from build123d import *

# Parameters (mm, degrees)
F1_DEPTH  = 101.6
F3_W      = 51.8218297699
F3_H      = 127
F4_DEPTH  = 88.9
F2_W      = 50.8
F2_H      = 127
F5_DEPTH  = 88.9
F7_DEPTH  = 76.2
F9_DEPTH  = 76.2
F11_DEPTH = 203.2
F13_DEPTH = 406.4


with BuildPart() as f1:
    # F0 (on Front) → F1 (new body, symmetric)
    with BuildSketch(Plane.XZ):
        Polygon((-63.5, 255.5875), (-203.2, 255.5875), (-167.3808159173, -1.6199540129), (-203.2, -14.6044082429), (-203.2, -255.5875), (203.2, -255.5875), (203.2, -14.6044082429), (167.3808159173, -1.6199540129), (203.2, 255.5875), (63.5, 255.5875), (63.5, 113.3475), (-63.5, 113.3475), align=None)
        Polygon((-63.5, 306.22875), (-203.2, 255.5875), (-63.5, 255.5875), align=None)
        Polygon((63.5, 306.22875), (63.5, 255.5875), (203.2, 255.5875), align=None)
        Polygon((203.2, -255.5875), (-203.2, -255.5875), (5.2712307392, -288.1220414472), align=None)
        Polygon((5.2712307392, -288.1220414472), (-203.2, -255.5875), (-203.2, -322.3895), align=None)
        Polygon((203.2, -319.0113), (203.2, -255.5875), (5.2712307392, -288.1220414472), align=None)
        Polygon((5.2712307392, -288.1220414472), (-203.2, -322.3895), (-203.2, -512.662041116), (6.3136153163, -545.3592597063), (203.2, -512.9960602239), (203.2, -319.0113), align=None)
        Polygon((6.3136153163, -545.3592597063), (-203.2, -512.662041116), (-203.2, -579.7980602239), align=None)
        Polygon((203.2, -576.085841116), (203.2, -512.9960602239), (6.3136153163, -545.3592597063), align=None)
        Polygon((6.3136153163, -545.3592597063), (-203.2, -579.7980602239), (-203.2, -814.3875), (203.2, -814.3875), (203.2, -576.085841116), align=None)
    extrude(amount=F1_DEPTH, both=True)

    # F3 (on face) → F4 (cut)
    with BuildSketch(Plane(origin=(-203.2, 0, 0), x_dir=(0, -1, 0), z_dir=(-1, 0, 0))):
        with Locations((-0.2844144409, 61.8800459871)):
            Rectangle(F3_W, F3_H)
    extrude(amount=-F4_DEPTH, mode=Mode.SUBTRACT)

    # F2 (on face) → F5 (cut)
    with BuildSketch(Plane.YZ.offset(203.2)):
        with Locations((-0.2265004441, 61.8800459871)):
            Rectangle(F2_W, F2_H)
    extrude(amount=-F5_DEPTH, mode=Mode.SUBTRACT)

    # F6 (on face) → F7 (cut)
    with BuildSketch(Plane.XZ.offset(101.6)):
        Polygon((203.2, -282.1055948734), (-203.2, -349.0782082081), (-203.2, -606.9228053093), (203.2, -539.9501919746), align=None)
    extrude(amount=-F7_DEPTH, mode=Mode.SUBTRACT)

    # F8 (on face) → F9 (cut)
    with BuildSketch(Plane(origin=(0, 101.6, 0), x_dir=(-1, 0, 0), z_dir=(0, 1, 0))):
        Polygon((-203.2, -346.3322222233), (-203.2, -603.5153269768), (203.2, -539.219558239), (203.2, -282.6924920082), align=None)
    extrude(amount=-F9_DEPTH, mode=Mode.SUBTRACT)

    # F10 (on face) → F11 (cut)
    with BuildSketch(Plane.XZ.offset(101.6)):
        Polygon((203.2, -776.2875), (165.1, -814.3875), (203.2, -814.3875), align=None)
        Polygon((-203.2, -814.3875), (-165.1, -814.3875), (-203.2, -776.2875), align=None)
    extrude(amount=-F11_DEPTH, mode=Mode.SUBTRACT)

    # F12 (on face) → F13 (cut)
    with BuildSketch(Plane.YZ.offset(203.2)):
        Polygon((-63.5, -814.3875), (-101.6, -776.2875), (-101.6029715538, -814.3875), align=None)
        Polygon((101.6, -814.3875), (101.6, -776.2875), (63.5, -814.3875), align=None)
    extrude(amount=-F13_DEPTH, mode=Mode.SUBTRACT)


solid = f1.part
Geometry: final body of the model. Coordinates: model frame, mm. A direction names the side the tool comes from. Coordinates: 2 decimals unless noted, no trailing zeros. Loops run counter-clockwise (first coordinate to the right, second up) from the corner with the lowest first, then second, coordinate; pieces in that order, holes last. Notation, with made-up numbers: M 5,-17 L 41,-17 A23 cw 41,2 Z; hole C 12,72 d7. An arc over 180 degrees is marked long. One line per item, written item: value. Start each with the question number.
1) Cut plane A-A (y = -5.5). Return loops of the section in (x, z), then the cut area to 3 significant figures.
2) Reachability of faces 4 (the flat face through (-185.04, -1.42, -8.02)), 5 (the flat face through (-2.845, -64.033, -573.905)), 6 (the flat face through (142, 25.173, 61)), 7 (the flat face through (-150, 1, 125.38)), 8 (the flat face through (-3, -25.4, -442)) from +Z, -Z, +X, -X, +Y, -Y: full face, straight path, thin tool, end or side. Return the list, or none.
3) Cut plane C-C (y = -75.5). Return loops of the section in (x, z).
4) Cut plane D-D (x = -10). Return loops of the section in (y, z), then the cut area to 3 significant figures.
5) Cut plane B-B (x = 124). Return loops of the section in (y, z).
6) Pin query (flat end, axial travel): P1, Ø1, axis at x = -115, z = -475.5, coming from the -Y side; P2, Ø2, axis at x = 137, y = 30.5, coming from the +Z side; P3, Ø1, axis at x = 52.5, y = -15.5, coming from the +Z side. Return the tip coordinate at first contact, or that it passes through.
7) Draft query along Z for faces 1 (the flat face through (-183.883, -1.422, -795.604)), 2 (the flat face through (-3, -101.6, -17)), 3 (the flat face through (142, -25.627, 61)). Return one class per face: released by +Z, released by -Z, zero draft, split by the parting line, or undercut.
8) Material intervals for L1, parallel to Z at x = -60, y = -45; L2, parallel to Z at x = 27, y = 83; L3, parallel to Z at x = -6.5, y = 8, sorted ascending. Write a range as from..to.
Evaluation:
1. outline: M -203.2,-776.29 L -165.1,-814.39 L 165.1,-814.39 L 203.2,-776.29 L 203.2,-14.6 L 167.38,-1.62 L 114.3,-1.62 L 114.3,125.38 L 185.07,125.38 L 203.2,255.59 L 63.5,306.23 L 63.5,113.35 L -63.5,113.35 L -63.5,306.23 L -203.2,255.59 L -185.07,125.38 L -114.3,125.38 L -114.3,-1.62 L -167.38,-1.62 L -203.2,-14.6 Z
1. area: 397,000 mm^2
2. face 4: -X, +Y, -Y
2. face 5: -X, -Y
2. face 6: +X
2. face 7: -X
2. face 8: -Y
3. outline: M -203.2,-776.29 L -177.1,-802.39 L 177.1,-802.39 L 203.2,-776.29 L 203.2,-539.95 L -203.2,-606.92 Z; M -203.2,-349.08 L 203.2,-282.11 L 203.2,-14.6 L 167.38,-1.62 L 203.2,255.59 L 63.5,306.23 L 63.5,113.35 L -63.5,113.35 L -63.5,306.23 L -203.2,255.59 L -167.38,-1.62 L -203.2,-14.6 Z
4. outline: M -101.6,-776.29 L -63.5,-814.39 L 63.5,-814.39 L 101.6,-776.29 L 101.6,-569.79 L 25.4,-569.79 L 25.4,-312.95 L 101.6,-312.95 L 101.6,113.35 L -101.6,113.35 L -101.6,-317.24 L -25.4,-317.24 L -25.4,-575.08 L -101.6,-575.08 Z
4. area: 148,000 mm^2
5. outline: M -101.6,-776.29 L -63.5,-814.39 L 63.5,-814.39 L 101.6,-776.29 L 101.6,-590.99 L 25.4,-590.99 L 25.4,-333.93 L 101.6,-333.93 L 101.6,284.3 L -101.6,284.3 L -101.6,-295.16 L -25.4,-295.16 L -25.4,-553 L -101.6,-553 Z; hole M -25.63,-1.62 L 25.17,-1.62 L 25.17,125.38 L -25.63,125.38 Z
6. P1: y = -25.4
6. P2: z = 279.95
6. P3: z = 113.35
7. face 1: released by -Z
7. face 2: zero draft
7. face 3: undercut
8. L1: -814.39..-583.32, -325.48..113.35
8. L2: -794.89..-575.64, -318.74..113.35
8. L3: -814.39..113.35
